Input: part model. Units: mm. Frame: model coordinates. A direction names the side the tool comes from. Round coordinates to 2 decimals unless told otherwise and drop trailing zeros. Write each loop counter-clockwise with the first axis right and the second up, starting at its lowest first coordinate (ties: lowest second). Pieces come first, ordered by that corner, then holes. Notation, with made-up numbers: M -26.5,71 L -9.5,71 A32 ccw -9.5,101 Z; hole C 4.25,-35.5 d4. An arc over 180 degrees is marked long. Answer as CSV lines item,"result". Start each with the question number.
```python
from build123d import *

# Parameters (mm, degrees)
FILLET1_R = 2


with BuildPart() as part:
    # Sketch1 → Revolve1 (revolve)
    with BuildSketch(Plane(origin=(0, 0, 0), x_dir=(1, 0, 0), z_dir=(0, 1, 0)), mode=Mode.PRIVATE) as revolve1_sk:
        Polygon((0, 51.25), (0, 55.5), (32, 55.5), (32, 58), (538, 58), (538, 55.5), (570, 55.5), (570, 51.25), (565.25, 50), (4.75, 50), align=None)
    revolve(revolve1_sk.sketch.rotate(Axis((0, 0, 0), (1, 0, 0)), 180), axis=Axis((0, 0, 0), (1, 0, 0)))

    # Fillet1
    fillet1_edges = [part.edges().sort_by_distance(p)[0] for p in [
        (32, 0, -55.5),
        (538, 0, -55.5),
    ]]
    fillet(fillet1_edges, radius=FILLET1_R)


solid = part.part
```
Item 1: Line query: line 1 (Y direction, x = 201, z = 0); line 2 (Y direction, x = 302.5, z = 35). Output: solid intervals per line, ascending. Write a range as [from, to].
Item 2: Pin query (flat end, axial travel): pin 1 Ø2 at (x, z) = (241.5, 11) entering from +Y; pin 2 Ø3 at (x, y) = (84.5, 14.5) entering from +Z; pin 3 Ø4 at (x, z) = (504.5, -6.5) entering from +Y. Return the tip coordinate at first contact, or that it passes through.
Item 3: Cut plane A-A, the plane y = 0. Return loops of the section in (x, z).
Item 4: Cut plane C-C, the plane x = 256. Return loops of the section in (y, z), plus the area to 3 significant figures.
Item 5: Access query for faces 5 (the face through (32, -51.8, -25.5)), 6 (the face through (555.21, -16.671, 52.937)), 7 (the face through (0, 16, -49)). Directions: +Z, -Z, +X, -X, +Y, -Y. A direction counts if a zero-diameter tool reaches every point of the face in a straight line with its end or side. Return the directions, or none.
Item 6: Draft query along Z for faces 1 (the face through (281.08, -15.02, 47.69)), 2 (the face through (4.45, 44.43, 23.11)), 3 (the face through (15.21, -16.671, 52.937)), 4 (the face through (538, 25.5, -51.8)). Return one class per face: +Z half, -Z half, draft (parallel to the pull), parting line (faces both ways), or undercut.
Results list:
1,line 1,"[-58, -50], [50, 58]"
1,line 2,"[-46.25, -35.71], [35.71, 46.25]"
2,pin 1,"y = 57.13"
2,pin 2,"z = 56.52"
2,pin 3,"y = 57.83"
3,outline,"M 0,-55.5 L 30,-55.5 A2 cw 32,-57.5 L 32,-58 L 538,-58 L 538,-57.5 A2 cw 540,-55.5 L 570,-55.5 L 570,-51.25 L 565.25,-50 L 4.75,-50 L 0,-51.25 Z; M 0,51.25 L 4.75,50 L 565.25,50 L 570,51.25 L 570,55.5 L 540,55.5 A2 cw 538,57.5 L 538,58 L 32,58 L 32,57.5 A2 cw 30,55.5 L 0,55.5 Z"
4,outline,"C 0,0 d116; hole C 0,0 d100"
4,area,"2,710 mm²"
5,face 5,"-X"
5,face 6,"+X"
5,face 7,"+Z, -Z, -X, +Y, -Y"
6,face 1,"undercut"
6,face 2,"undercut"
6,face 3,"parting line"
6,face 4,"draft"
